Geometry check sheet. Reference: the model listing, model coordinates, mm. A direction names the side the tool comes from. Give positions to 0.01 mm unless a question says otherwise; leave off trailing zeros. Write each loop counter-clockwise with the first axis right and the second up, starting at its lowest first coordinate (ties: lowest second). Pieces come first, ordered by that corner, then holes. Notation, with made-up numbers: (78, 45.25) -> (88, 45.25) arc R12 ccw to (88, 65.25) -> close; hole circle Ø7 at (55.5, 58). An arc over 180 degrees is marked (long way). One line per item, written item: value.
from build123d import *

# Parameters (mm, degrees)
SKETCH1_W           = 15
SKETCH1_H           = 15
SKETCH1_W_2         = 12
SKETCH1_H_2         = 12
EXTRUDE_THIN1_DEPTH = 356
SKETCH2_R           = 1.5
CUT_EXTRUDE1_DEPTH  = 357.631462437
SKETCH3_R           = 1.5
CUT_EXTRUDE2_DEPTH  = 357.631462437


with BuildPart() as part:
    # Sketch1 → Extrude-Thin1 (new body)
    with BuildSketch(Plane(origin=(0, 0, 0), x_dir=(1, 0, 0), z_dir=(0, 1, 0))):
        with Locations((7.5, 7.5)):
            Rectangle(SKETCH1_W, SKETCH1_H)
        with Locations((7.5, 7.5)):
            Rectangle(SKETCH1_W_2, SKETCH1_H_2, mode=Mode.SUBTRACT)
    extrude(amount=EXTRUDE_THIN1_DEPTH)

    # Sketch2 (on Front Plane) → Cut-Extrude1 (cut, through all)
    with BuildSketch(Plane.XY):
        with Locations((7.5, 27.5)):
            Circle(SKETCH2_R)
        with Locations((7.5, 47.5)):
            Circle(SKETCH2_R)
        with Locations((7.5, 42.5)):
            Circle(SKETCH2_R)
        with Locations((7.5, 328.5)):
            Circle(SKETCH2_R)
        with Locations((7.5, 313.5)):
            Circle(SKETCH2_R)
        with Locations((7.5, 308.5)):
            Circle(SKETCH2_R)
    extrude(amount=-CUT_EXTRUDE1_DEPTH, mode=Mode.SUBTRACT)

    # Sketch3 → Cut-Extrude2 (cut, through all)
    with BuildSketch(Plane(origin=(15, 0, 0), x_dir=(0, 0, -1), z_dir=(1, 0, 0))):
        with Locations((7.5, 276.148)):
            Circle(SKETCH3_R)
        with Locations((7.5, 256.148)):
            Circle(SKETCH3_R)
        with Locations((7.5, 198)):
            Circle(SKETCH3_R)
        with Locations((7.5, 158)):
            Circle(SKETCH3_R)
        with Locations((7.5, 99.852)):
            Circle(SKETCH3_R)
        with Locations((7.5, 79.852)):
            Circle(SKETCH3_R)
    extrude(amount=-CUT_EXTRUDE2_DEPTH, mode=Mode.SUBTRACT)


solid = part.part
1) Sectioned sample at A-A on y = 55. Record the cut outline in (x, z), plus the area to 3 significant figures.
Verdict:
outline: (0, -15) -> (15, -15) -> (15, 0) -> (0, 0) -> close; hole (1.5, -13.5) -> (13.5, -13.5) -> (13.5, -1.5) -> (1.5, -1.5) -> close
area: 81.0 mm^2
2) Tool access check on faces 4 (the flat face through (0, 176, -7)), 5 (the flat face through (1.5, 176, -7)). Record the directions out of +Z, -Z, +X, -X, +Y, -Y that give a thin tool (end or side, any length) a straight path to the whole face; none if there is none.
Verdict:
face 4: +Z, -Z, -X, +Y, -Y
face 5: +Y, -Y
3) Mould release check, pull along Z, two halves, no side actions. Record for faces 1 (the flat face through (14, 0, -8)), 2 (the flat face through (7, 176, -15)), 3 (the flat face through (7, 176, -1.5)): released by +Z, released by -Z, zero draft, split by the parting line, or undercut.
Verdict:
face 1: zero draft
face 2: released by -Z
face 3: undercut
4) Scan lines: probe 1 along X at (y, z) = (203, -4); probe 2 along Z at (x, y) = (3, 63); probe 3 along Z at (x, y) = (14.15, 158). Record each from-to range of solid material in increasing order.
Verdict:
probe 1: 0 to 1.5, 13.5 to 15
probe 2: -15 to -13.5, -1.5 to 0
probe 3: -15 to -9, -6 to 0
5) Depth check by flat-ended pin: pin 1 Ø4 at (x, y) = (9.5, 214.5) entering from +Z. Enter the tip coordinate at first touch or a pass-through.
Verdict:
pin 1: z = 0
